from build123d import *

# Parameters (mm, degrees)
F0_W   = 134.5115825534
F0_H   = 15.5633129179
F0_W_2 = 25.5161747336
F0_H_2 = 18.5351353139
F0_W_3 = 23.8279551268
F0_H_3 = 15.50362329


with BuildPart() as f1:
    # F0 (on Front) → F1 (revolve)
    with BuildSketch(Plane.XZ):
        with Locations((-5.3299926221, 11.8945706636)):
            Rectangle(F0_W, F0_H)
        Polygon((69.2527592182, 29.1677135974), (69.2527592182, 47.7028489113), (61.9257986546, 47.7028489113), (61.9257986546, 19.6762271225), (61.9257986546, 4.1129142046), (61.9257986546, -19.2015636712), (69.2527592182, -19.2015636712), (69.2527592182, -3.6979403812), align=None)
        with Locations((82.010846585, 38.4352812544)):
            Rectangle(F0_W_2, F0_H_2)
        with Locations((81.1667367816, -11.4497520262)):
            Rectangle(F0_W_3, F0_H_3)
    revolve(axis=Axis((-72.5857838988, 0, 11.8945706636), (0, 0, -1)))


solid = f1.part
Build history of the part. All positions in model axes, mm. A direction names the side the tool comes from. Coordinates: 2 decimals unless noted, no trailing zeros. Write each loop counter-clockwise with the first axis right and the second up, starting at its lowest first coordinate (ties: lowest second). Pieces come first, ordered by that corner, then holes. Notation, with made-up numbers: (31.5, 3) -> (35.5, 3) arc R14 ccw to (35.5, 21) -> close; hole circle Ø5 at (64, 34.5). An arc over 180 degrees is marked (long way). Use CSV: the item, a comma, the result in double quotes. Start each with the question number.
Q1. Cut at C-C, the plane x = 30.5. List the corners of the cut face in (y, z).
Q2. Drill centre lines: probe 1 along X at (y, z) = (0, 35.75); probe 2 along Z at (x, y) = (-168.5, -110.5); probe 3 along X at (y, z) = (0, -9.25). Where is each one in solid material? Low to high.
Q3. 3-axis set-ups, long thin cutter, end or side, ignore diameter. For faces 1 (the cylindrical face through (87.04, -50.27, 38.57)), 2 (the flat face through (-72, -136, -19.202)), 3 (the flat face through (-195, -74, -3.698)), 4 (the flat face through (-71, -2, 4.113)), 5 (the cylindrical face through (-206.967, -5.914, 33.493)): which of +Z, -Z, +X, -X, +Y, -Y reach the whole face in a straight line?
Q4. Pull direction X, two halves, no side cores. Call faces 6 (the flat face through (-71, -2, 19.676)), 7 (the flat face through (65, -38, 29.168)), 8 (the cylindrical face through (-238.092, -7.284, -11.341)): released by +X, released by -X, zero draft, split by the parting line, or undercut.
Q5. Cut at A-A, the plane y = 0. List the corners of the cut face in (x, z), then the cut area to 3 significant figures.
Q6. Flat gauge pins, fed straight in: pin 1 Ø1.5 at (x, z) = (8.5, 32.5) entering from +Y; pin 2 Ø12 at (y, z) = (34.5, -3.5) entering from +X; pin 3 Ø4 at (x, z) = (-114.5, 40) entering from +Y. Where does each tip first touch, or does it go through?
Q7. Cut at B-B, the plane y = -147. List the corners of the cut face in (x, z).
Checked values:
1,outline,"(-131.84, 29.17) -> (-97.42, 29.17) -> (-97.42, -3.7) -> (-129.69, -3.7) -> (-129.69, -19.2) -> (-86.41, -19.2) -> (-86.41, 4.11) -> (86.41, 4.11) -> (86.41, -19.2) -> (129.69, -19.2) -> (129.69, -3.7) -> (97.42, -3.7) -> (97.42, 29.17) -> (131.84, 29.17) -> (131.84, 47.7) -> (86.41, 47.7) -> (86.41, 19.68) -> (-86.41, 19.68) -> (-86.41, 47.7) -> (-131.84, 47.7) -> close"
2,probe 1,"x = -239.94 to -207.1, 61.93 to 94.77"
2,probe 2,"z = -19.2 to -3.7, 29.17 to 47.7"
2,probe 3,"x = -238.25 to -207.1, 61.93 to 93.08"
3,face 1,"+Z, -Z"
3,face 2,"-Z, +X, -X, +Y, -Y"
3,face 3,"none"
3,face 4,"-Z"
3,face 5,"+Z"
4,face 6,"undercut"
4,face 7,"zero draft"
4,face 8,"split by the parting line"
5,outline,"(-239.94, 29.17) -> (-214.42, 29.17) -> (-214.42, -3.7) -> (-238.25, -3.7) -> (-238.25, -19.2) -> (-207.1, -19.2) -> (-207.1, 4.11) -> (61.93, 4.11) -> (61.93, -19.2) -> (93.08, -19.2) -> (93.08, -3.7) -> (69.25, -3.7) -> (69.25, 29.17) -> (94.77, 29.17) -> (94.77, 47.7) -> (61.93, 47.7) -> (61.93, 19.68) -> (-207.1, 19.68) -> (-207.1, 47.7) -> (-239.94, 47.7) -> close"
5,area,"6,850 mm²"
6,pin 1,"stops at y = 146.81"
6,pin 2,"stops at x = 90.61"
6,pin 3,"stops at y = 162.53"
7,outline,"(-152.58, 29.17) -> (7.41, 29.17) -> (7.41, 47.7) -> (-152.58, 47.7) -> close; (-148.98, -19.2) -> (3.81, -19.2) -> (3.81, -3.7) -> (-148.98, -3.7) -> close"
